The model under review builds one solid part; all positions refer to its coordinate system, in mm. A direction names the side the tool comes from. Coordinates: 2 decimals unless noted, no trailing zeros. Order: outer loops, then holes, each group sorted by start corner. A loop starts at its lowest first (then second) coordinate and runs counter-clockwise, first axis right, second up.
from build123d import *

# Parameters (mm, degrees)
SKETCH_2_R      = 1.5
SKETCH_2_R_2    = 1.6
SKETCH_2_R_3    = 1.75
SKETCH_2_R_4    = 9
SKETCH_2_R_5    = 10
EXTRUDE_1_DEPTH = 5


with BuildPart() as part:
    # 草图2 → 凸台-拉伸1 (new body)
    with BuildSketch(Plane.XY):
        with BuildLine():
            Line((-165.542218516, 84.933067874), (84.457781484, 84.933067874))
            ThreePointArc((84.457781484, 84.933067874), (91.528849296, 82.004135686), (94.457781484, 74.933067874))
            Line((94.457781484, 74.933067874), (94.457781484, -75.066932126))
            ThreePointArc((94.457781484, -75.066932126), (91.528849296, -82.137999937), (84.457781484, -85.066932126))
            Line((84.457781484, -85.066932126), (-165.542218516, -85.066932126))
            ThreePointArc((-165.542218516, -85.066932126), (-172.613286328, -82.137999937), (-175.542218516, -75.066932126))
            Line((-175.542218516, -75.066932126), (-175.542218516, 74.933067874))
            ThreePointArc((-175.542218516, 74.933067874), (-172.613286328, 82.004135686), (-165.542218516, 84.933067874))
        make_face()
        with Locations((-145.542218516, 72.933067874)):
            Circle(SKETCH_2_R, mode=Mode.SUBTRACT)
        with Locations((-115.542218516, 72.933067874)):
            Circle(SKETCH_2_R, mode=Mode.SUBTRACT)
        with Locations((-146.065799187, 48.933067874)):
            Circle(SKETCH_2_R, mode=Mode.SUBTRACT)
        with Locations((-116.065799187, 48.933067874)):
            Circle(SKETCH_2_R, mode=Mode.SUBTRACT)
        with Locations(Location((-116.065799187, -49.066932126, 0), (0, 0, 180))):
            Circle(SKETCH_2_R, mode=Mode.SUBTRACT)
        with Locations(Location((-115.542218516, -73.066932126, 0), (0, 0, 180))):
            Circle(SKETCH_2_R, mode=Mode.SUBTRACT)
        with Locations(Location((-145.542218516, -73.066932126, 0), (0, 0, 180))):
            Circle(SKETCH_2_R, mode=Mode.SUBTRACT)
        with Locations(Location((-146.065799187, -49.066932126, 0), (0, 0, 180))):
            Circle(SKETCH_2_R, mode=Mode.SUBTRACT)
        with Locations(Location((64.981362155, 48.933067874, 0), (0, 0, 180))):
            Circle(SKETCH_2_R, mode=Mode.SUBTRACT)
        with Locations(Location((34.981362155, 48.933067874, 0), (0, 0, 180))):
            Circle(SKETCH_2_R, mode=Mode.SUBTRACT)
        with Locations(Location((34.457781484, 72.933067874, 0), (0, 0, 180))):
            Circle(SKETCH_2_R, mode=Mode.SUBTRACT)
        with Locations(Location((64.457781484, 72.933067874, 0), (0, 0, 180))):
            Circle(SKETCH_2_R, mode=Mode.SUBTRACT)
        with Locations((34.457781484, -73.066932126)):
            Circle(SKETCH_2_R, mode=Mode.SUBTRACT)
        with Locations((34.981362155, -49.066932126)):
            Circle(SKETCH_2_R, mode=Mode.SUBTRACT)
        with Locations((64.981362155, -49.066932126)):
            Circle(SKETCH_2_R, mode=Mode.SUBTRACT)
        with Locations((64.457781484, -73.066932126)):
            Circle(SKETCH_2_R, mode=Mode.SUBTRACT)
        with Locations((74.457781484, 37.433067874)):
            Circle(SKETCH_2_R_2, mode=Mode.SUBTRACT)
        with Locations(Location((74.457781484, -37.566932126, 0), (0, 0, 180))):
            Circle(SKETCH_2_R_2, mode=Mode.SUBTRACT)
        with Locations((69.457781484, 4.933067874)):
            Circle(SKETCH_2_R_2, mode=Mode.SUBTRACT)
        with Locations((21.457781484, 4.933067874)):
            Circle(SKETCH_2_R_2, mode=Mode.SUBTRACT)
        with Locations(Location((69.457781484, -5.066932126, 0), (0, 0, 180))):
            Circle(SKETCH_2_R_2, mode=Mode.SUBTRACT)
        with Locations(Location((21.457781484, -5.066932126, 0), (0, 0, 180))):
            Circle(SKETCH_2_R_2, mode=Mode.SUBTRACT)
        with Locations((-23.944476924, -29.764734827)):
            Circle(SKETCH_2_R_3, mode=Mode.SUBTRACT)
        with Locations((-51.884476924, -29.764734827)):
            Circle(SKETCH_2_R_3, mode=Mode.SUBTRACT)
        with Locations((-8.704476924, 21.035265173)):
            Circle(SKETCH_2_R_3, mode=Mode.SUBTRACT)
        with Locations((-56.964476924, 22.305265173)):
            Circle(SKETCH_2_R_3, mode=Mode.SUBTRACT)
        with Locations((2.799841961, -0.066932126)):
            Circle(SKETCH_2_R_4, mode=Mode.SUBTRACT)
        with Locations((-80.295672717, -0.066932126)):
            Circle(SKETCH_2_R_4, mode=Mode.SUBTRACT)
        with Locations((-160.542218516, 60.933067874)):
            Circle(SKETCH_2_R_5, mode=Mode.SUBTRACT)
        with Locations(Location((-160.542218516, -61.066932126, 0), (0, 0, 180))):
            Circle(SKETCH_2_R_5, mode=Mode.SUBTRACT)
        with Locations((-77.330354065, -56.066932126)):
            Circle(SKETCH_2_R_2, mode=Mode.SUBTRACT)
        with Locations((-77.330354065, -77.066932126)):
            Circle(SKETCH_2_R_2, mode=Mode.SUBTRACT)
        with Locations((3.229701528, -48.443032681)):
            Circle(SKETCH_2_R_2, mode=Mode.SUBTRACT)
        with Locations((79.457781484, -61.066932126)):
            Circle(SKETCH_2_R_5, mode=Mode.SUBTRACT)
        with Locations(Location((79.457781484, 60.933067874, 0), (0, 0, 180))):
            Circle(SKETCH_2_R_5, mode=Mode.SUBTRACT)
        with BuildLine():
            Line((-157.542218516, 34.913165474), (-157.542218516, -35.047029725))
            ThreePointArc((-157.542218516, -35.047029725), (-160.542218516, -38.047029725), (-163.542218516, -35.047029725))
            Line((-163.542218516, -35.047029725), (-163.542218516, 34.913165474))
            ThreePointArc((-163.542218516, 34.913165474), (-160.542218516, 37.913165474), (-157.542218516, 34.913165474))
        make_face(mode=Mode.SUBTRACT)
        with BuildLine():
            Line((-132.542218516, 34.913165474), (-132.542218516, -35.047029725))
            ThreePointArc((-132.542218516, -35.047029725), (-135.542218516, -38.047029725), (-138.542218516, -35.047029725))
            Line((-138.542218516, -35.047029725), (-138.542218516, 34.913165474))
            ThreePointArc((-138.542218516, 34.913165474), (-135.542218516, 37.913165474), (-132.542218516, 34.913165474))
        make_face(mode=Mode.SUBTRACT)
        with BuildLine():
            Line((-107.542218516, 34.913165474), (-107.542218516, -35.047029725))
            ThreePointArc((-107.542218516, -35.047029725), (-110.542218516, -38.047029725), (-113.542218516, -35.047029725))
            Line((-113.542218516, -35.047029725), (-113.542218516, 34.913165474))
            ThreePointArc((-113.542218516, 34.913165474), (-110.542218516, 37.913165474), (-107.542218516, 34.913165474))
        make_face(mode=Mode.SUBTRACT)
        with BuildLine():
            ThreePointArc((-95.414503132, -37.564666946), (-40.542218516, -49.29309446), (14.330066101, -37.564666946))
            ThreePointArc((14.330066101, -37.564666946), (16.597243532, -31.618247309), (10.650823895, -29.351069878))
            ThreePointArc((10.650823895, -29.351069878), (-40.542218516, -40.29309446), (-91.735260926, -29.351069878))
            ThreePointArc((-91.735260926, -29.351069878), (-97.681680563, -31.618247309), (-95.414503132, -37.564666946))
        make_face(mode=Mode.SUBTRACT)
        with BuildLine():
            ThreePointArc((-95.414503132, 37.430802695), (-40.542218516, 49.159230209), (14.330066101, 37.430802695))
            ThreePointArc((14.330066101, 37.430802695), (16.597243532, 31.484383058), (10.650823895, 29.217205627))
            ThreePointArc((10.650823895, 29.217205627), (-40.542218516, 40.159230209), (-91.735260926, 29.217205627))
            ThreePointArc((-91.735260926, 29.217205627), (-97.681680563, 31.484383058), (-95.414503132, 37.430802695))
        make_face(mode=Mode.SUBTRACT)
    extrude(amount=EXTRUDE_1_DEPTH)


solid = part.part
(1) Tool access review of faces 5 (the face through (-41.33, -49.29, 2.46)), 6 (the face through (-39, 1, 0)): name each direction out of +Z, -Z, +X, -X, +Y, -Y from which nothing blocks a thin tool from reaching the whole face with its end or side.
(2) The part is to be moulded in two halves that separate along Y. For faces 1 (the face through (-175.542, -1, 2)), 2 (the face through (-39.804, 40.157, 2.465)), 3 (the face through (-163.542, -1, 2)), 4 (the face through (-39, -85.067, 2)), say which applies: +Y half, -Y half, draft (parallel to the pull), parting line (faces both ways), or undercut.
(3) Consider section B-B (x = -1.5). Give the boundary of the cut face in (y, z), then the cut area to 3 significant figures.
(4) Consider section A-A (y = 16.5). Give the boundary of the cut face in (x, z).
(5) Wall thickness on line 1 (Y direction, x = -38, z = 1.1); line 2 (X direction, y = 12, z = 2.2); line 3 (X direction, y = 0.5, z = 2.65): over which ranges is each line inside the solid? List them lowest first.
(6) Consider section D-D (x = -154.5). Give the boundary of the cut face in (y, z), then the cut area to 3 significant figures.
(7) Consider section C-C (y = -68.5). Give the boundary of the cut face in (x, z).
Findings:
1. face 5: +Z, -Z
1. face 6: -Z, +X, -X, +Y, -Y
2. face 1: draft
2. face 2: undercut
2. face 3: undercut
2. face 4: -Y half
3. outline: (-85.07, 0) - (-43.49, 0) - (-43.49, 5) - (-85.07, 5) - close; (-34.05, 0) - (-7.97, 0) - (-7.97, 5) - (-34.05, 5) - close; (7.84, 0) - (33.92, 0) - (33.92, 5) - (7.84, 5) - close; (43.36, 0) - (84.93, 0) - (84.93, 5) - (43.36, 5) - close
3. area: 677 mm2
4. outline: (-175.54, 0) - (-163.54, 0) - (-163.54, 5) - (-175.54, 5) - close; (-157.54, 0) - (-138.54, 0) - (-138.54, 5) - (-157.54, 5) - close; (-132.54, 0) - (-113.54, 0) - (-113.54, 5) - (-132.54, 5) - close; (-107.54, 0) - (94.46, 0) - (94.46, 5) - (-107.54, 5) - close
5. line 1: y = -85.07 to -49.27, -40.27 to 40.13, 49.14 to 84.93
5. line 2: x = -175.54 to -163.54, -157.54 to -138.54, -132.54 to -113.54, -107.54 to 94.46
5. line 3: x = -175.54 to -163.54, -157.54 to -138.54, -132.54 to -113.54, -107.54 to -89.28, -71.31 to -6.18, 11.78 to 94.46
6. outline: (-85.07, 0) - (-69.04, 0) - (-69.04, 5) - (-85.07, 5) - close; (-53.1, 0) - (52.96, 0) - (52.96, 5) - (-53.1, 5) - close; (68.9, 0) - (84.93, 0) - (84.93, 5) - (68.9, 5) - close
6. area: 691 mm2
7. outline: (-175.54, 0) - (-167.23, 0) - (-167.23, 5) - (-175.54, 5) - close; (-153.85, 0) - (72.77, 0) - (72.77, 5) - (-153.85, 5) - close; (86.15, 0) - (94.46, 0) - (94.46, 5) - (86.15, 5) - close
